from build123d import *

# Parameters (mm, degrees)
SKETCH_1_W      = 47.8
SKETCH_1_H      = 6.7
EXTRUDE_1_DEPTH = 5
CHAMFER_1_SIZE  = 0.5


with BuildPart() as part:
    # Эскиз1 → Бобышка-Вытянуть1 (new body)
    with BuildSketch(Plane(origin=(0, 66.754264805, 0), x_dir=(-1, 0, 0), z_dir=(0, 0, 1))):
        with Locations((0, 66.654264805)):
            Rectangle(SKETCH_1_W, SKETCH_1_H)
        Polygon((-20.9, 67.204264805), (-20.9, 66.304264805), (20.9, 66.304264805), (20.9, 67.204264805), (12.5, 67.204264805), (11.75, 68.504264805), (11, 67.204264805), (-11, 67.204264805), (-11.75, 68.504264805), (-12.5, 67.204264805), align=None, mode=Mode.SUBTRACT)
    extrude(amount=EXTRUDE_1_DEPTH)

    # Фаска1
    chamfer_1_edges = [part.edges().sort_by_distance(p)[0] for p in [
        (16.7, -0.45, 5),
        (20.9, 0, 5),
        (0, 0.45, 5),
        (-20.9, 0, 5),
        (-16.7, -0.45, 5),
        (0, -0.45, 5),
    ]]
    chamfer(chamfer_1_edges, length=CHAMFER_1_SIZE)


solid = part.part
Build history of the part. All positions in model axes, mm. A direction names the side the tool comes from. Give positions to 0.01 mm unless a question says otherwise; leave off trailing zeros. Order: outer loops, then holes, each group sorted by start corner. A loop starts at its lowest first (then second) coordinate and runs counter-clockwise, first axis right, second up. Notation, with made-up numbers: M 88.5,35.5 L 109.5,35.5 A20 ccw 109.5,39.5 Z; hole C 66,-4 d10. An arc over 180 degrees is marked long. Put each result on its own line as item: value.
Item 1: Slice it at B-B, the plane y = 0. Write the cut outline in (x, z), plus the area to 4 significant figures.
From the geometry:
outline: M -23.9,0 L -20.9,0 L -20.9,4.5 L -21.4,5 L -23.9,5 Z; M 20.9,0 L 23.9,0 L 23.9,5 L 21.4,5 L 20.9,4.5 Z
area: 29.75 mm2
Item 2: Two-plate mould, pull along Y, no slides. Class faces 3 (the flat face through (0, -0.45, 2)), 4 (the flat face through (0, 3.45, 2)), 5 (the flat face through (12.12, -1.11, 2.46)), 6 (the flat face through (23.9, 0, 2)): +Y half, -Y half, draft (parallel to the pull), parting line (faces both ways), or undercut.
From the geometry:
face 3: undercut
face 4: +Y half
face 5: undercut
face 6: draft
Item 3: Slice it at A-A, the plane x = -5.5. Write the cut outline in (y, z).
From the geometry:
outline: M -3.25,0 L -0.45,0 L -0.45,4.5 L -0.95,5 L -3.25,5 Z; M 0.45,0 L 3.45,0 L 3.45,5 L 0.95,5 L 0.45,4.5 Z
Item 4: Slice it at C-C, the plane z = 3.05. Write the cut outline in (x, y).
From the geometry:
outline: M -23.9,-3.25 L 23.9,-3.25 L 23.9,3.45 L -23.9,3.45 Z; hole M -20.9,-0.45 L -12.5,-0.45 L -11.75,-1.75 L -11,-0.45 L 11,-0.45 L 11.75,-1.75 L 12.5,-0.45 L 20.9,-0.45 L 20.9,0.45 L -20.9,0.45 Z
Item 5: Probe line 1 (Y direction, x = 5, z = 2.1); line 2 (X direction, y = 0, z = 4.15); line 3 (X direction, y = -0.75, z = 4.6). List the from-to ranges inside material, lowest first. Write a range as [from, to].
From the geometry:
line 1: y = [-3.25, -0.45], [0.45, 3.45]
line 2: x = [-23.9, -20.9], [20.9, 23.9]
line 3: x = [-23.9, -12.33], [-11.17, 11.17], [12.33, 23.9]
Item 6: 3-axis set-ups, long thin cutter, end or side, ignore diameter. For faces 1 (the flat face through (0, 2, 5)), 2 (the flat face through (0, 0.45, 2)): which of +Z, -Z, +X, -X, +Y, -Y reach the whole face in a straight line?
From the geometry:
face 1: +Z, +X, -X, +Y, -Y
face 2: +Z, -Z
